Answer from the drawing. Dimensions are ordinates in mm from the lowest x, y and z of the part. A direction names the side the tool comes from. Round coordinates to 2 decimals unless told otherwise and drop trailing zeros. Order: outer loops, then holes, each group sorted by start corner. A loop starts at its lowest first (then second) coordinate and runs counter-clockwise, first axis right, second up. Notation, with made-up numbers: (-14.75, 82) -> (24.25, 82) arc R17 cw to (24.25, 98) -> close; hole circle Ø1 at (-5.5, 2.5). An arc over 180 degrees is marked (long way). Use a Markdown table: item, result. Add a question column.
1. Consider L1, parallel to Y at x = 5.5, z = 5.65; L2, parallel to Z at x = 1, y = 4.75; L3, parallel to Y at x = 5, z = 4.9. Determine where each line is inside the solid, lowest interval first. Write a range as [from, to].
2. Given pin 1 (5 mm diameter, centred on x = 5.5, y = 6.5, fed in from +Z); pin 2 (0.5 mm diameter, centred on x = 3, y = 2, fed in from -Z); pin 3 (2 mm diameter, centred on x = 9, z = 1.5, fed in from +Y); pin 4 (1 mm diameter, centred on x = 5.5, y = 7.5, fed in from +Z), each flat-ended and moving along its own axis, determine where each tip first touches the part or whether it passes through.
3. For the marked faces 4 and 5, determine the directions among +Z, -Z, +X, -X, +Y, -Y from which every point of the face is accessible in a straight line to the end or side of a thin tool.
4. Section B-B, the plane y = 5.75 is taken. Give the vertices of the cut face in (x, z), then the cut area to 3 significant figures.
5. Section D-D, the plane y = 0.5 is taken. Give the vertices of the cut face in (x, z), then the cut area to 3 significant figures.
6. The mould has two halves that part along X. Classify the marked faces 1, 2 and 3: +X half, -X half, draft (parallel to the pull), parting line (faces both ways), or undercut.
7. Section C-C, the plane x = 4.75 is taken. Give the vertices of the cut face in (y, z), then the cut area to 3 significant figures.
8. Section A-A, the plane z = 5.5 is taken. Give the vertices of the cut face in (x, y), then the cut area to 3 significant figures.
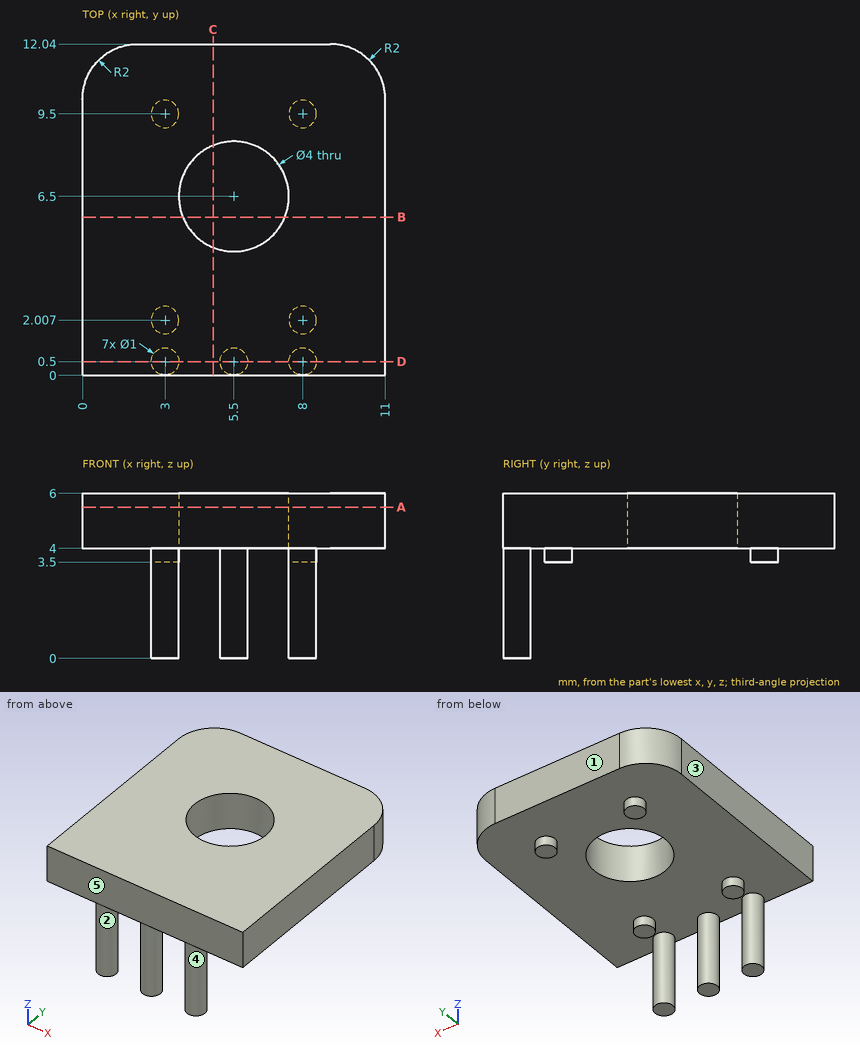
Verdict:
| question | item | result |
|---|---|---|
| 1 | L1 | y = [0, 4.5], [8.5, 12.04] |
| 1 | L2 | z = [4, 6] |
| 1 | L3 | y = [0, 4.56], [8.44, 12.04] |
| 2 | pin 1 | stops at z = 6 |
| 2 | pin 2 | stops at z = 3.5 |
| 2 | pin 3 | stops at y = 1 |
| 2 | pin 4 | passes through |
| 3 | face 4 | -Z |
| 3 | face 5 | +Z, -Z, +X, -X, -Y |
| 4 | outline | (0, 4) -> (3.65, 4) -> (3.65, 6) -> (0, 6) -> close; (7.35, 4) -> (11, 4) -> (11, 6) -> (7.35, 6) -> close |
| 4 | area | 14.6 mm2 |
| 5 | outline | (0, 4) -> (2.5, 4) -> (2.5, 0) -> (3.5, 0) -> (3.5, 4) -> (5, 4) -> (5, 0) -> (6, 0) -> (6, 4) -> (7.5, 4) -> (7.5, 0) -> (8.5, 0) -> (8.5, 4) -> (11, 4) -> (11, 6) -> (0, 6) -> close |
| 5 | area | 34.0 mm2 |
| 6 | face 1 | draft |
| 6 | face 2 | undercut |
| 6 | face 3 | -X half |
| 7 | outline | (0, 4) -> (4.65, 4) -> (4.65, 6) -> (0, 6) -> close; (8.35, 4) -> (12.04, 4) -> (12.04, 6) -> (8.35, 6) -> close |
| 7 | area | 16.7 mm2 |
| 8 | outline | (0, 0) -> (11, 0) -> (11, 10.04) arc R2 ccw to (9, 12.04) -> (2, 12.04) arc R2 ccw to (0, 10.04) -> close; hole circle Ø4 at (5.5, 6.5) |
| 8 | area | 118 mm2 |
